```python
from build123d import *

# Parameters (mm, degrees)
SKETCH1_W           = 125
SKETCH1_H           = 76.2
BOSS_EXTRUDE1_DEPTH = 3
SKETCH2_W           = 3
SKETCH2_H           = 76.2
BOSS_EXTRUDE2_DEPTH = 22
SKETCH4_W           = 25
SKETCH4_H           = 4
BOSS_EXTRUDE4_DEPTH = 21.59
SKETCH5_W           = 25
SKETCH5_H           = 4
BOSS_EXTRUDE5_DEPTH = 21.59
SKETCH6_W           = 168.18
SKETCH6_H           = 25.4
BOSS_EXTRUDE6_DEPTH = 3
CHAMFER1_SIZE       = 28
SKETCH7_W           = 93.6
SKETCH7_H           = 26
CUT_EXTRUDE1_DEPTH  = 2
SKETCH9_W           = 119
SKETCH9_H           = 3
BOSS_EXTRUDE7_DEPTH = 22
CHAMFER2_SIZE       = 4
CHAMFER3_SIZE       = 5
CUT_EXTRUDE2_START  = -0.6
CUT_EXTRUDE2_DEPTH  = 0.6
SKETCH11_R          = 1.75
CUT_EXTRUDE3_DEPTH  = 5
FILLET1_R           = 1
CHAMFER4_SIZE       = 1.5


# Read off the part's stored shape, not the designer's step: Cut-Extrude2
with BuildPart() as part:
    # Sketch1 → Boss-Extrude1 (new body)
    with BuildSketch(Plane.XY):
        Rectangle(SKETCH1_W, SKETCH1_H)
    extrude(amount=BOSS_EXTRUDE1_DEPTH)

    # Sketch2 → Boss-Extrude2 (add)
    with BuildSketch(Plane.XY.offset(3)):
        with Locations((-61, 0)):
            Rectangle(SKETCH2_W, SKETCH2_H)
        with Locations((61, 0)):
            Rectangle(SKETCH2_W, SKETCH2_H)
    extrude(amount=BOSS_EXTRUDE2_DEPTH)

    # Sketch4 → Boss-Extrude4 (add)
    with BuildSketch(Plane.ZY.offset(62.5)):
        with Locations((12.5, 36.1)):
            Rectangle(SKETCH4_W, SKETCH4_H)
    extrude(amount=BOSS_EXTRUDE4_DEPTH)

    # Sketch5 → Boss-Extrude5 (add)
    with BuildSketch(Plane(origin=(62.5, 0, 0), x_dir=(0, 0, -1), z_dir=(1, 0, 0))):
        with Locations((-12.5, 36.1)):
            Rectangle(SKETCH5_W, SKETCH5_H)
    extrude(amount=BOSS_EXTRUDE5_DEPTH)

    # Sketch6 → Boss-Extrude6 (add)
    with BuildSketch(Plane(origin=(0, 0, 0), x_dir=(-1, 0, 0), z_dir=(0, 0, -1))):
        with Locations((0, 50.8)):
            Rectangle(SKETCH6_W, SKETCH6_H)
    extrude(amount=-BOSS_EXTRUDE6_DEPTH)

    # Chamfer1
    chamfer1_edges = [part.edges().sort_by_distance(p)[0] for p in [
        (-84.09, 63.5, 1.5),
        (84.09, 63.5, 1.5),
    ]]
    chamfer(chamfer1_edges, length=CHAMFER1_SIZE)

    # Sketch7 → Cut-Extrude1 (cut)
    with BuildSketch(Plane.XY.offset(3)):
        with Locations((0, -9.4)):
            Rectangle(SKETCH7_W, SKETCH7_H)
        with Locations((0, 36.6)):
            Rectangle(SKETCH7_W, SKETCH7_H)
    extrude(amount=-CUT_EXTRUDE1_DEPTH, mode=Mode.SUBTRACT)

    # Sketch9 → Boss-Extrude7 (add)
    with BuildSketch(Plane.XY.offset(3)):
        with Locations((0, -36.6)):
            Rectangle(SKETCH9_W, SKETCH9_H)
    extrude(amount=BOSS_EXTRUDE7_DEPTH)

    # Chamfer2
    chamfer2_edges = [part.edges().sort_by_distance(p)[0] for p in [
        (-59.5, -35.1, 14),
        (59.5, -35.1, 14),
    ]]
    chamfer(chamfer2_edges, length=CHAMFER2_SIZE)

    # Chamfer3
    chamfer3_edges = [part.edges().sort_by_distance(p)[0] for p in [
        (62.5, -38.1, 12.5),
        (-62.5, -38.1, 12.5),
    ]]
    chamfer(chamfer3_edges, length=CHAMFER3_SIZE)

    # Cut-Extrude2 outline → Cut-Extrude2 (cut)
    # profile 1 of 4: a face of its own
    with BuildSketch(Plane.XY.offset(3).offset(CUT_EXTRUDE2_START)):
        with BuildLine():
            Line((-12.843793417, 16.784775128), (-13.918894641, 13.722312614))
            add(Edge.make_bspline(
                [(-13.918894641, 13.722312614), (-13.950745906, 13.608646354), (-13.97919001, 13.483685694), (-14.011317489, 13.235305925), (-14.01541758, 13.110841548), (-13.989547543, 12.867284383), (-13.959604678, 12.747961158), (-13.857332343, 12.519974586), (-13.78490702, 12.411398187), (-13.592313629, 12.212018271), (-13.472083062, 12.121314997), (-13.184369222, 11.962818623), (-13.016909084, 11.895027419), (-12.454211206, 11.728033285), (-11.997806272, 11.664794493), (-11.025815686, 11.62704002), (-10.511530183, 11.651603075), (-9.78258436, 11.770518687), (-9.546683753, 11.824200176), (-9.102156978, 11.962599668), (-8.89364967, 12.047436893), (-8.514064046, 12.246658938), (-8.343153207, 12.361026326), (-8.04132547, 12.611058926), (-7.910418089, 12.746448479), (-7.679883041, 13.0275306), (-7.579636344, 13.172799488), (-7.44297026, 13.39668043), (-7.39971151, 13.472431032), (-7.318663078, 13.627460279), (-7.280772846, 13.706786212), (-7.248185858, 13.788667895)],
                knots=[0, 0, 0, 0, 0.0625, 0.0625, 0.125, 0.125, 0.1875, 0.1875, 0.25, 0.25, 0.3125, 0.3125, 0.375, 0.375, 0.5, 0.5, 0.625, 0.625, 0.6875, 0.6875, 0.75, 0.75, 0.8125, 0.8125, 0.875, 0.875, 0.9375, 0.9375, 0.96875, 0.96875, 1, 1, 1, 1], degree=3))
            Line((-7.248185858, 13.788667895), (-6.196379448, 16.784775128))
            Line((-6.196379448, 16.784775128), (-7.771512854, 16.784775171))
            Line((-7.771512854, 16.784775171), (-8.779640442, 13.913087848))
            add(Edge.make_bspline(
                [(-8.779640442, 13.913087848), (-8.801212863, 13.867686768), (-8.828630281, 13.811426743), (-8.890437912, 13.684919137), (-8.925723343, 13.615289873), (-9.014867696, 13.477778317), (-9.069034752, 13.410065742), (-9.20356673, 13.286811644), (-9.283951715, 13.231246188), (-9.470687062, 13.136081945), (-9.576947425, 13.096402347), (-9.809000897, 13.032201026), (-9.934689567, 13.00760449), (-10.326953956, 12.952228061), (-10.607716868, 12.939250309), (-11.138236784, 12.940792557), (-11.387946526, 12.95495502), (-11.815776289, 13.010911905), (-11.994686961, 13.05312605), (-12.19022456, 13.154353945), (-12.243244201, 13.194586759), (-12.322270156, 13.289978248), (-12.348136332, 13.345299657), (-12.373130151, 13.46826163), (-12.371956966, 13.5361378), (-12.35254935, 13.67085438), (-12.333771283, 13.737944141), (-12.322165603, 13.788667937)],
                knots=[0, 0, 0, 0, 0.0625, 0.0625, 0.125, 0.125, 0.1875, 0.1875, 0.25, 0.25, 0.3125, 0.3125, 0.375, 0.375, 0.5, 0.5, 0.625, 0.625, 0.75, 0.75, 0.8125, 0.8125, 0.875, 0.875, 0.9375, 0.9375, 1, 1, 1, 1], degree=3))
            Line((-12.322165603, 13.788667937), (-11.2703582, 16.784775128))
            Line((-11.2703582, 16.784775128), (-12.843793417, 16.784775128))
        make_face()
    # profile 2 of 4: a face of its own
    with BuildSketch(Plane.XY.offset(3).offset(CUT_EXTRUDE2_START)):
        Polygon((14.082145905, 15.466432145), (14.547318434, 16.784775128), (8.481425261, 16.784775128), (8.015662645, 15.45803385), (10.386127447, 15.45803385), (9.075451111, 11.743439605), (10.661733364, 11.743439605), (11.975372051, 15.466432145), align=None)
    # profile 3 of 4: a face of its own
    with BuildSketch(Plane.XY.offset(3).offset(CUT_EXTRUDE2_START)):
        Polygon((0.359928822, 15.45803385), (0.825593089, 16.784775128), (-5.237786258, 16.784775128), (-5.705919648, 15.45803385), (-3.328357423, 15.45803385), (-4.639000977, 11.723834147), (-3.059652234, 11.723834147), (-1.74900868, 15.45803385), align=None)
    # profile 4 of 4: a face of its own
    with BuildSketch(Plane.XY.offset(3).offset(CUT_EXTRUDE2_START)):
        Polygon((7.732615088, 18.009820452), (8.67993853, 22.298690548), (4.451236342, 18.010625114), (-13.617285872, 18.010625114), (-13.760696138, 17.631800344), (4.083976363, 17.631800344), (-2.561139847, 10.89339914), (-16.036862666, 10.89339914), (-16.175076152, 10.505618026), (-2.943552817, 10.505618026), (-8.264964605, 5.10950355), (-0.819885517, 10.505618026), (5.569839691, 10.505618026), (5.813932632, 9.32327198), (6.07620201, 10.510665049), (13.482070183, 10.510665049), (13.624063348, 10.89339914), (6.160742258, 10.89339914), (7.649117922, 17.631800344), (15.972876762, 17.631800344), (16.113123511, 18.009820452), align=None)
        Polygon((-0.283933962, 10.894070437), (4.780674194, 14.564845582), (5.489286994, 10.894070437), align=None, mode=Mode.SUBTRACT)
        Polygon((5.863139247, 17.323666682), (5.364033793, 14.945937564), (5.179256414, 15.9244998), (2.885975157, 14.289472868), align=None, mode=Mode.SUBTRACT)
    extrude(amount=CUT_EXTRUDE2_DEPTH, mode=Mode.SUBTRACT)

    # Sketch11 → Cut-Extrude3 (cut)
    with BuildSketch(Plane(origin=(0, 38.1, 0), x_dir=(1, 0, 0), z_dir=(0, 1, 0))):
        with Locations(Location((-76.11, -13, 0), (0, 0, 270))):
            Circle(SKETCH11_R)
        with Locations(Location((76.29, -13, 0), (0, 0, 270))):
            Circle(SKETCH11_R)
    extrude(amount=-CUT_EXTRUDE3_DEPTH, mode=Mode.SUBTRACT)

    # Fillet1
    fillet1_edges = [part.edges().sort_by_distance(p)[0] for p in [
        (-62.5, 34.1, 12.5),
        (62.5, 34.1, 12.5),
    ]]
    fillet(fillet1_edges, radius=FILLET1_R)

    # Chamfer4
    chamfer4_edges = [part.edges().sort_by_distance(p)[0] for p in [
        (-59.5, 38.1, 14),
        (59.5, 38.1, 14),
    ]]
    chamfer(chamfer4_edges, length=CHAMFER4_SIZE)


solid = part.part
```
Can you work these out from the model? Positions are in its coordinate system, mm. A direction names the side the tool comes from. Give positions to 0.01 mm unless a question says otherwise; leave off trailing zeros. Order: outer loops, then holes, each group sorted by start corner. A loop starts at its lowest first (then second) coordinate and runs counter-clockwise, first axis right, second up. Notation, with made-up numbers: (36.5, -28.5) - (93.5, -28.5) arc R29 cw to (93.5, -8.5) - close; hole circle Ø1 at (13, 49). An arc over 180 degrees is marked (long way). Use a Markdown table: item, result. Add a question column.
Q1. If we mould it in two halves opening along Z, with no side actions, what happens to faces 1 (the cylindrical face through (74.58, 36.13, 12.62)), 2 (the flat face through (1, 15, 3)), 3 (the flat face through (60, -35.6, 12.3))? For each: released by +Z, released by -Z, zero draft, split by the parting line, or undercut.
Q2. Please list where these lines run through material, in increasing order: line 1 along Y through (x, z) = (-8.5, 2); line 2 along X through (y, z) = (3, 13); line 3 along Z through (x, y) = (76.29, 35.2).
Q3. I'm going to push flat-ended pins straight in: pin 1 (8 mm diameter, centred on y = -5.5, z = 9.5, fed in from -X); pin 2 (12.5 mm diameter, centred on y = 4, z = 14, fed in from +X); pin 3 (8 mm diameter, centred on x = 1, y = -13.5, fed in from +Z); pin 4 (8 mm diameter, centred on y = 44, z = 11, fed in from +X). Where does each tip first touch, or does it pass through?
Q4. If we section it at B-B on z = 13: Count the separate pieces of the cut face and the enclosed holes in it, plus the area to 3 significant figures.
Q5. On a 3-axis mill with a long thin cutter (end or side, diameter ignored), from which of +Z, -Z, +X, -X, +Y, -Y can I reach the whole of each face in a straight line? I mean faces 4 (the flat face through (-1, -35.1, 14)), 5 (the flat face through (-1, -9, 1)), 6 (the flat face through (74, 34.1, 13)). Say none if no direction works.
Q6. If we section it at D-D on y = -26: Write out the boundary of the cut face in (x, z), plus the area to 3 significant figures.
Q7. If we section it at C-C on x = 18.5: Write out the boundary of the cut face in (y, z), plus the area to 3 significant figures.
Q8. If we section it at A-A on x = -76.11: Write out the boundary of the cut face in (y, z).
Answers follow:
| question | item | result |
|---|---|---|
| 1 | face 1 | undercut |
| 1 | face 2 | released by +Z |
| 1 | face 3 | zero draft |
| 2 | line 1 | y = -38.1 to -22.4, 3.6 to 23.6, 49.6 to 63.5 |
| 2 | line 2 | x = -62.5 to -59.5, 59.5 to 62.5 |
| 2 | line 3 | z = 0 to 11.25, 14.75 to 25 |
| 3 | pin 1 | stops at x = -62.5 |
| 3 | pin 2 | stops at x = 62.5 |
| 3 | pin 3 | stops at z = 1 |
| 3 | pin 4 | passes through |
| 4 | separate pieces | 3 |
| 4 | enclosed holes | 0 |
| 4 | area | 941 mm^2 |
| 5 | face 4 | +Z, +Y |
| 5 | face 5 | +Z |
| 5 | face 6 | +Z, -Z, +X, -Y |
| 6 | outline | (-62.5, 0) - (62.5, 0) - (62.5, 25) - (59.5, 25) - (59.5, 3) - (-59.5, 3) - (-59.5, 25) - (-62.5, 25) - close |
| 6 | area | 507 mm^2 |
| 7 | outline | (-38.1, 0) - (63.5, 0) - (63.5, 3) - (49.6, 3) - (49.6, 1) - (23.6, 1) - (23.6, 3) - (3.6, 3) - (3.6, 1) - (-22.4, 1) - (-22.4, 3) - (-35.1, 3) - (-35.1, 25) - (-38.1, 25) - close |
| 7 | area | 267 mm^2 |
| 8 | outline | (34.1, 0) - (43.48, 0) - (43.48, 3) - (38.1, 3) - (38.1, 11.25) - (34.1, 11.25) - close; (34.1, 14.75) - (38.1, 14.75) - (38.1, 25) - (34.1, 25) - close |
